```python
from build123d import *

# Parameters (mm, degrees)
ESBO_O2_R                         = 11.4
RESSALTO_EXTRUS_O3_DEPTH          = 7
ESBO_O1_R                         = 2.4
CORTE_EXTRUS_O4_DEPTH             = 15
ESBO_O6_R                         = 3.9
RESSALTO_EXTRUS_O5_DEPTH          = 2
CORTE_EXTRUS_O7_DEPTH             = 4
CORTE_EXTRUS_O7_DEPTH_BACK        = 6
ESBO_O4_R                         = 2
CORTE_EXTRUS_O8_DEPTH             = 10.5
CORTE_EXTRUS_O9_REACH             = 23.588
ESBO_O8_R                         = 1.5
CORTE_EXTRUS_O9_DIRECTION_2_DEPTH = 22.588411189


with BuildPart() as part:
    # Esboço2 → Ressalto-extrusão3 (new body)
    with BuildSketch(Plane(origin=(0, 0, 0), x_dir=(1, 0, 0), z_dir=(0, 1, 0))):
        with Locations(Location((0, 0, 0), (0, 0, 270))):
            Circle(ESBO_O2_R)
    extrude(amount=RESSALTO_EXTRUS_O3_DEPTH)

    # Esboço1 → Corte-extrusão4 (cut)
    with BuildSketch(Plane(origin=(0, 0, 0), x_dir=(1, 0, 0), z_dir=(0, 1, 0))):
        with Locations(Location((-6.59, 3.46, 0), (0, 0, 270))):
            Circle(ESBO_O1_R)
        with Locations(Location((6.59, -3.46, 0), (0, 0, 90))):
            Circle(ESBO_O1_R)
        with Locations(Location((0, -8, 0), (0, 0, 90))):
            Circle(ESBO_O1_R)
        with Locations(Location((-6.59, -3.46, 0), (0, 0, 90))):
            Circle(ESBO_O1_R)
    extrude(amount=CORTE_EXTRUS_O4_DEPTH, mode=Mode.SUBTRACT)

    # Esboço6 → Ressalto-extrusão5 (add)
    with BuildSketch(Plane.XZ):
        with Locations(Location((0, 0, 0), (0, 0, 90))):
            Circle(ESBO_O6_R)
    extrude(amount=RESSALTO_EXTRUS_O5_DEPTH)

    # Esboço4 → Corte-extrusão7 (cut, two sides: drawn at the far end of the back side and taken through both)
    with BuildSketch(Plane(origin=(0, 0, 0), x_dir=(-1, 0, 0), z_dir=(0, -1, 0)).offset(-CORTE_EXTRUS_O7_DEPTH_BACK)):
        with Locations(Location((0, 0, 0), (0, 0, 90))):
            Circle(ESBO_O4_R)
    extrude(amount=CORTE_EXTRUS_O7_DEPTH + CORTE_EXTRUS_O7_DEPTH_BACK, mode=Mode.SUBTRACT)

    # Esboço7 → Corte-extrusão8 (cut)
    with BuildSketch(Plane.XZ):
        Polygon((7.212489168, -2.828427125), (2.828427125, -7.212489168), (0.848528137, -5.232590181), (3.040559159, -3.040559159), (5.232590181, -0.848528137), align=None)
    extrude(amount=-CORTE_EXTRUS_O8_DEPTH, mode=Mode.SUBTRACT)

    # Esboço8 → Corte-extrusão9 (cut, up to next)
    with BuildSketch(Plane(origin=(3.040559159, 0, -3.040559159), x_dir=(-0.7071067811865475, 0, -0.7071067811865477), z_dir=(0.7071067811865477, 0, -0.7071067811865475)), mode=Mode.PRIVATE) as corte_extrus_o9_sk1:
        with Locations((0, 3.5)):
            Circle(ESBO_O8_R)
    corte_extrus_o9_tool1 = extrude(corte_extrus_o9_sk1.sketch, amount=-CORTE_EXTRUS_O9_REACH, mode=Mode.PRIVATE) & part.part
    add(corte_extrus_o9_tool1.solids().sort_by_distance((3.040559, 3.5, -3.040559))[0], mode=Mode.SUBTRACT)

    # Esboço8 → Corte-extrusão9 direction 2 (cut)
    with BuildSketch(Plane(origin=(3.040559159, 0, -3.040559159), x_dir=(-0.7071067811865475, 0, -0.7071067811865477), z_dir=(0.7071067811865477, 0, -0.7071067811865475))):
        with Locations((0, 3.5)):
            Circle(ESBO_O8_R)
    extrude(amount=CORTE_EXTRUS_O9_DIRECTION_2_DEPTH, mode=Mode.SUBTRACT)


solid = part.part
```
Model file for the job. Use its own axes, mm. A direction names the side the tool comes from. Round coordinates to 2 decimals unless told otherwise and drop trailing zeros. Order: outer loops, then holes, each group sorted by start corner. A loop starts at its lowest first (then second) coordinate and runs counter-clockwise, first axis right, second up. Notation, with made-up numbers: M -2,72 L 2,72 A10 ccw 2,89 Z; hole C 85.5,20 d2. An arc over 180 degrees is marked long. Use CSV: the item, a comma, the result in double quotes.
Item 1: Saw through at C-C (z = 3.46). List the corners of the cut face in (x, y), plus the area to 3 significant figures.
Worked answers:
outline,"M -10.86,0 L -8.99,0 L -8.99,7 L -10.86,7 Z; M -4.19,0 L -1.8,0 L -1.8,-2 L 1.8,-2 L 1.8,0 L 4.19,0 L 4.19,7 L -4.19,7 Z; M 8.99,0 L 10.86,0 L 10.86,7 L 8.99,7 Z"
area,"92.1 mm²"
Item 2: Saw through at B-B (y = 1.25). List the corners of the cut face in (x, z), plus the area to 3 significant figures.
Worked answers:
outline,"C 0,0 d22.8; hole C -6.59,-3.46 d4.8; hole C -6.59,3.46 d4.8; hole C 0,8 d4.8; hole C 0,0 d4; hole M 0.85,-5.23 L 2.83,-7.21 L 7.21,-2.83 L 5.23,-0.85 Z; hole C 6.59,3.46 d4.8"
area,"306 mm²"
Item 3: Saw through at D-D (x = -3.25). List the corners of the cut face in (y, z), plus the area to 3 significant figures.
Worked answers:
outline,"M -2,-2.16 L 0,-2.16 L 0,-10.93 L 7,-10.93 L 7,10.93 L 0,10.93 L 0,2.16 L -2,2.16 Z"
area,"162 mm²"
Item 4: Which spindle directions (+Z, -Z, +X, -X, +Y, -Y) get a long thin tool onto all of the face, cutting with end or side? Do faces 5 (the face through (2.373, -0.986, -3.095)), 6 (the face through (7.58, 3.57, -5.46)), 7 (the face through (6.209, 3.451, -1.825)). Say none if no direction does.
Worked answers:
face 5,"-Y"
face 6,"none"
face 7,"+Y, -Y"
Item 5: Pin check, flat tips, straight feed: pin 1 (6 mm diameter, centred on x = 0.5, z = 5, fed in from -Y); pin 2 (4 mm diameter, centred on x = 0, z = 8, fed in from -Y); pin 3 (5.5 mm diameter, centred on x = 6.59, z = 3.46, fed in from -Y); pin 4 (4 mm diameter, centred on y = 6, z = 8, fed in from +X). Stop position of each tip, or through.
Worked answers:
pin 1,"y = -2"
pin 2,"through"
pin 3,"y = 0"
pin 4,"x = 9.69"
Item 6: Pull direction X, two halves, no side cores. Call faces 1 (the face through (-8.933, 3.451, -3.98)), 2 (the face through (-4.37, 3.45, 10.53)), 3 (the face through (0, 0, -5)), 4 (the face through (-1.2, 2.1, 1.6)): released by +X, released by -X, zero draft, split by the parting line, or undercut.
Worked answers:
face 1,"undercut"
face 2,"split by the parting line"
face 3,"zero draft"
face 4,"undercut"
Item 7: Saw through at A-A (x = -6.59). List the corners of the cut face in (y, z).
Worked answers:
outline,"M 0,-9.3 L 7,-9.3 L 7,-5.86 L 0,-5.86 Z; M 0,-1.06 L 7,-1.06 L 7,1.06 L 0,1.06 Z; M 0,5.86 L 7,5.86 L 7,9.3 L 0,9.3 Z"
Item 8: Probe probe 1 along X at (y, z) = (3.25, -6.5); probe 2 along X at (y, z) = (5, -3.46); probe 3 along X at (y, z) = (1, 0). List the from-to ranges inside material, lowest first.
Worked answers:
probe 1,"-9.37 to 2.12, 3.54 to 4.41, 8.59 to 9.37"
probe 2,"-10.86 to -8.99, -4.19 to 2.62, 6.58 to 10.86"
probe 3,"-11.4 to -2, 2 to 11.4"
